Read the model definition and answer for the solid it produces. Units are mm, in the model's axes. A direction names the side the tool comes from. Give positions to 0.01 mm unless a question says otherwise; leave off trailing zeros. Order: outer loops, then holes, each group sorted by start corner. A loop starts at its lowest first (then second) coordinate and runs counter-clockwise, first axis right, second up. Notation, with made-up numbers: (-23, 14.5) - (17, 14.5) arc R17 ccw to (17, 47.5) - close; hole circle Ø6 at (20.5, 42). An arc over 180 degrees is marked (long way). Write item = value, one per line.
```python
from build123d import *

# Parameters (mm, degrees)
SKETCH3_R           = 43
SKETCH3_R_2         = 20
BOSS_EXTRUDE1_DEPTH = 25


with BuildPart() as part:
    # Sketch1 → Revolve1 (revolve)
    with BuildSketch(Plane(origin=(0, 0, 0), x_dir=(1, 0, 0), z_dir=(0, 1, 0))):
        Polygon((0, -75), (45, -75), (45, -175), (25, -175), (25, -820.014288631), (0, -820.014288631), align=None)
    revolve(axis=Axis((0, 0, 75), (0, 0, 1)))

    # Sketch3 → Boss-Extrude1 (add, symmetric)
    with BuildSketch(Plane(origin=(0, 0, 0), x_dir=(1, 0, 0), z_dir=(0, 1, 0))):
        with Locations((0, -855)):
            Circle(SKETCH3_R)
        with Locations((0, -855)):
            Circle(SKETCH3_R_2, mode=Mode.SUBTRACT)
    extrude(amount=BOSS_EXTRUDE1_DEPTH, both=True)


solid = part.part
```
1. Straight lines are drawn through the part: L1, parallel to Z at x = 0, y = -10; L2, parallel to X at y = -4, z = 855; L3, parallel to Z at x = -22, y = 32. For each, find the intervals that lie inside material, in ascending order. Write a range as [from, to].
Recorded:
L1 = [75, 835], [875, 898]
L2 = [-43, -20], [20, 43]
L3 = [75, 175]
2. Determine the mould class of faces 3 (the face through (23.846, 7.509, 502.023)), 4 (the face through (1, 1, 75)), 5 (the face through (9, 25, 874)), 6 (the face through (-2.6, -0.35, 835.17)) for opening direction Z: +Z half, -Z half, draft (parallel to the pull), parting line (faces both ways), or undercut.
Recorded:
face_3 = undercut
face_4 = -Z half
face_5 = draft
face_6 = undercut
3. Section D-D (y = -32.5) is taken. Determine the outline of the cut face in (x, z).
Recorded:
outline = (-31.12, 75) - (31.12, 75) - (31.12, 175) - (-31.12, 175) - close
4. Section B-B (y = 0) is taken. Determine the outline of the cut face in (x, z), and give its area (3 significant figures).
Recorded:
outline = (-45, 75) - (45, 75) - (45, 175) - (25, 175) - (25, 820.01) arc R43 ccw (long way) to (-25, 820.01) - (-25, 175) - (-45, 175) - close; hole circle Ø40 at (0, 855)
area = 45,500 mm^2
5. Section C-C (z = 606.5) is taken. Determine the outline of the cut face in (x, y), and give its area (3 significant figures).
Recorded:
outline = circle Ø50 at (0, 0)
area = 1,960 mm^2
6. For faces 1 (the face through (9, -25, 874)), 2 (the face through (19, -19, 175)), determine the directions among +Z, -Z, +X, -X, +Y, -Y from which every point of the face is accessible in a straight line to the end or side of a thin tool.
Recorded:
face_1 = +Z, +X, -X, -Y
face_2 = none
7. Flat-ended cylindrical pins translate along their axes: pin 1 (6 mm diameter, centred on x = 10, z = 459.5, fed in from -Y); pin 2 (5 mm diameter, centred on y = -28, z = 372.5, fed in from -X); pin 3 (1.5 mm diameter, centred on x = 18, z = 481, fed in from -Y); pin 4 (4 mm diameter, centred on y = -7.5, z = 576.5, fed in from +X). Find the tip coordinate at first contact, or state that the pin passes through.
Recorded:
pin_1 = -24
pin_2 = through
pin_3 = -18.1
pin_4 = 24.39
8. Section A-A (z = 855) is taken. Determine the outline of the cut face in (x, y), and give its area (3 significant figures).
Recorded:
outline = (-43, -25) - (-20, -25) - (-20, 25) - (-43, 25) - close; (20, -25) - (43, -25) - (43, 25) - (20, 25) - close
area = 2,300 mm^2
